```python
from build123d import *

# Parameters (mm, degrees)
EXTRUDE_1_DEPTH     = 7
SKETCH_2_R          = 15
EXTRUDE_2_DEPTH     = 18.4
EXTRUDE_3_DEPTH     = 7
EXTRUDE_START       = 6.3
SKETCH_4_R          = 15
EXTRUDE_4_DEPTH     = 6.3
SKETCH_5_R          = 15
EXTRUDE_5_DEPTH     = 6.3
SKETCH_6_R          = 5
CUT_EXTRUDE_1_DEPTH = 90.291681756


with BuildPart() as part:
    # 草图1 → 凸台-拉伸1 (new body)
    with BuildSketch(Plane.XY.offset(28.9)):
        with BuildLine():
            Line((42.411201909, 45.77806603), (42.129389286, 47.376304833))
            ThreePointArc((42.129389286, 47.376304833), (40.514502568, 47.409839327), (38.89961585, 47.376304833))
            Line((38.89961585, 47.376304833), (38.617803227, 45.77806603))
            ThreePointArc((38.617803227, 45.77806603), (37.528159676, 43.541003491), (35.420005537, 42.219088972))
            ThreePointArc((35.420005537, 42.219088972), (32.937471152, 42.04939837), (30.741018632, 43.218743572))
            Line((30.741018632, 43.218743572), (29.573606233, 44.346100621))
            ThreePointArc((29.573606233, 44.346100621), (28.247424353, 43.424024), (26.960664635, 42.447687427))
            Line((26.960664635, 42.447687427), (27.672094632, 40.98903977))
            ThreePointArc((27.672094632, 40.98903977), (28.10546685, 38.538741749), (27.176936184, 36.230148526))
            ThreePointArc((27.176936184, 36.230148526), (25.268265311, 34.633668845), (22.80397403, 34.288646587))
            Line((22.80397403, 34.288646587), (21.196873713, 34.514509808))
            ThreePointArc((21.196873713, 34.514509808), (20.665953073, 32.989024), (20.198818833, 31.442812735))
            Line((20.198818833, 31.442812735), (21.631749371, 30.680910052))
            ThreePointArc((21.631749371, 30.680910052), (23.422603901, 28.95330711), (24.028363863, 26.539839327))
            ThreePointArc((24.028363863, 26.539839327), (23.422603901, 24.126371544), (21.631749371, 22.398768602))
            Line((21.631749371, 22.398768602), (20.198818833, 21.63686592))
            ThreePointArc((20.198818833, 21.63686592), (20.665953073, 20.090654655), (21.196873713, 18.565168847))
            Line((21.196873713, 18.565168847), (22.80397403, 18.791032067))
            ThreePointArc((22.80397403, 18.791032067), (25.268265311, 18.446009809), (27.176936184, 16.849530129))
            ThreePointArc((27.176936184, 16.849530129), (28.10546685, 14.540936905), (27.672094632, 12.090638884))
            Line((27.672094632, 12.090638884), (26.960664635, 10.631991228))
            ThreePointArc((26.960664635, 10.631991228), (28.247424353, 9.655654655), (29.573606233, 8.733578033))
            Line((29.573606233, 8.733578033), (30.741018632, 9.860935083))
            ThreePointArc((30.741018632, 9.860935083), (32.937471152, 11.030280285), (35.420005536, 10.860589683))
            ThreePointArc((35.420005536, 10.860589683), (37.528159676, 9.538675164), (38.617803227, 7.301612625))
            Line((38.617803227, 7.301612625), (38.89961585, 5.703373822))
            ThreePointArc((38.89961585, 5.703373822), (40.514502568, 5.669839327), (42.129389286, 5.703373822))
            Line((42.129389286, 5.703373822), (42.411201909, 7.301612625))
            ThreePointArc((42.411201909, 7.301612625), (43.50084546, 9.538675164), (45.6089996, 10.860589683))
            ThreePointArc((45.6089996, 10.860589683), (48.091533984, 11.030280285), (50.287986504, 9.860935083))
            Line((50.287986504, 9.860935083), (51.455398903, 8.733578033))
            ThreePointArc((51.455398903, 8.733578033), (52.781580783, 9.655654655), (54.068340501, 10.631991228))
            Line((54.068340501, 10.631991228), (53.356910504, 12.090638884))
            ThreePointArc((53.356910504, 12.090638884), (52.923538286, 14.540936905), (53.852068952, 16.849530129))
            ThreePointArc((53.852068952, 16.849530129), (55.760739826, 18.446009809), (58.225031106, 18.791032067))
            Line((58.225031106, 18.791032067), (59.832131424, 18.565168847))
            ThreePointArc((59.832131424, 18.565168847), (60.363052063, 20.090654655), (60.830186304, 21.63686592))
            Line((60.830186304, 21.63686592), (59.397255765, 22.398768602))
            ThreePointArc((59.397255765, 22.398768602), (57.606401235, 24.126371544), (57.000641274, 26.539839327))
            ThreePointArc((57.000641274, 26.539839327), (57.606401235, 28.95330711), (59.397255765, 30.680910052))
            Line((59.397255765, 30.680910052), (60.830186304, 31.442812735))
            ThreePointArc((60.830186304, 31.442812735), (60.363052063, 32.989024), (59.832131424, 34.514509808))
            Line((59.832131424, 34.514509808), (58.225031106, 34.288646587))
            ThreePointArc((58.225031106, 34.288646587), (55.760739826, 34.633668845), (53.852068952, 36.230148526))
            ThreePointArc((53.852068952, 36.230148526), (52.923538286, 38.538741749), (53.356910504, 40.98903977))
            Line((53.356910504, 40.98903977), (54.068340501, 42.447687427))
            ThreePointArc((54.068340501, 42.447687427), (52.781580783, 43.424024), (51.455398903, 44.346100621))
            Line((51.455398903, 44.346100621), (50.287986504, 43.218743572))
            ThreePointArc((50.287986504, 43.218743572), (48.091533984, 42.04939837), (45.6089996, 42.219088972))
            ThreePointArc((45.6089996, 42.219088972), (43.50084546, 43.541003491), (42.411201909, 45.77806603))
        make_face()
    extrude(amount=-EXTRUDE_1_DEPTH)

    # 草图2 → 凸台-拉伸2 (add)
    with BuildSketch(Plane(origin=(0, 0, 21.9), x_dir=(-1, 0, 0), z_dir=(0, 0, -1))):
        with Locations((-40.514502568, 26.539839327)):
            Circle(SKETCH_2_R)
    extrude(amount=EXTRUDE_2_DEPTH)

    # 草图3 → 凸台-拉伸3 (add)
    with BuildSketch(Plane.XY.offset(3.5)):
        with BuildLine():
            Line((42.411201909, 45.77806603), (42.129389286, 47.376304833))
            ThreePointArc((42.129389286, 47.376304833), (40.514502568, 47.409839327), (38.89961585, 47.376304833))
            Line((38.89961585, 47.376304833), (38.617803227, 45.77806603))
            ThreePointArc((38.617803227, 45.77806603), (37.528159676, 43.541003491), (35.420005537, 42.219088972))
            ThreePointArc((35.420005537, 42.219088972), (32.937471152, 42.04939837), (30.741018632, 43.218743572))
            Line((30.741018632, 43.218743572), (29.573606233, 44.346100621))
            ThreePointArc((29.573606233, 44.346100621), (28.247424353, 43.424024), (26.960664635, 42.447687427))
            Line((26.960664635, 42.447687427), (27.672094632, 40.98903977))
            ThreePointArc((27.672094632, 40.98903977), (28.10546685, 38.538741749), (27.176936184, 36.230148526))
            ThreePointArc((27.176936184, 36.230148526), (25.268265311, 34.633668845), (22.80397403, 34.288646587))
            Line((22.80397403, 34.288646587), (21.196873713, 34.514509808))
            ThreePointArc((21.196873713, 34.514509808), (20.665953073, 32.989024), (20.198818833, 31.442812735))
            Line((20.198818833, 31.442812735), (21.631749371, 30.680910052))
            ThreePointArc((21.631749371, 30.680910052), (23.422603901, 28.95330711), (24.028363863, 26.539839327))
            ThreePointArc((24.028363863, 26.539839327), (23.422603901, 24.126371544), (21.631749371, 22.398768602))
            Line((21.631749371, 22.398768602), (20.198818833, 21.63686592))
            ThreePointArc((20.198818833, 21.63686592), (20.665953073, 20.090654655), (21.196873713, 18.565168847))
            Line((21.196873713, 18.565168847), (22.80397403, 18.791032067))
            ThreePointArc((22.80397403, 18.791032067), (25.268265311, 18.446009809), (27.176936184, 16.849530129))
            ThreePointArc((27.176936184, 16.849530129), (28.10546685, 14.540936905), (27.672094632, 12.090638884))
            Line((27.672094632, 12.090638884), (26.960664635, 10.631991228))
            ThreePointArc((26.960664635, 10.631991228), (28.247424353, 9.655654655), (29.573606233, 8.733578033))
            Line((29.573606233, 8.733578033), (30.741018632, 9.860935083))
            ThreePointArc((30.741018632, 9.860935083), (32.937471152, 11.030280285), (35.420005536, 10.860589683))
            ThreePointArc((35.420005536, 10.860589683), (37.528159676, 9.538675164), (38.617803227, 7.301612625))
            Line((38.617803227, 7.301612625), (38.89961585, 5.703373822))
            ThreePointArc((38.89961585, 5.703373822), (40.514502568, 5.669839327), (42.129389286, 5.703373822))
            Line((42.129389286, 5.703373822), (42.411201909, 7.301612625))
            ThreePointArc((42.411201909, 7.301612625), (43.50084546, 9.538675164), (45.6089996, 10.860589683))
            ThreePointArc((45.6089996, 10.860589683), (48.091533984, 11.030280285), (50.287986504, 9.860935083))
            Line((50.287986504, 9.860935083), (51.455398903, 8.733578033))
            ThreePointArc((51.455398903, 8.733578033), (52.781580783, 9.655654655), (54.068340501, 10.631991228))
            Line((54.068340501, 10.631991228), (53.356910504, 12.090638884))
            ThreePointArc((53.356910504, 12.090638884), (52.923538286, 14.540936905), (53.852068952, 16.849530129))
            ThreePointArc((53.852068952, 16.849530129), (55.760739826, 18.446009809), (58.225031106, 18.791032067))
            Line((58.225031106, 18.791032067), (59.832131424, 18.565168847))
            ThreePointArc((59.832131424, 18.565168847), (60.363052063, 20.090654655), (60.830186304, 21.63686592))
            Line((60.830186304, 21.63686592), (59.397255765, 22.398768602))
            ThreePointArc((59.397255765, 22.398768602), (57.606401235, 24.126371544), (57.000641274, 26.539839327))
            ThreePointArc((57.000641274, 26.539839327), (57.606401235, 28.95330711), (59.397255765, 30.680910052))
            Line((59.397255765, 30.680910052), (60.830186304, 31.442812735))
            ThreePointArc((60.830186304, 31.442812735), (60.363052063, 32.989024), (59.832131424, 34.514509808))
            Line((59.832131424, 34.514509808), (58.225031106, 34.288646587))
            ThreePointArc((58.225031106, 34.288646587), (55.760739826, 34.633668845), (53.852068952, 36.230148526))
            ThreePointArc((53.852068952, 36.230148526), (52.923538286, 38.538741749), (53.356910504, 40.98903977))
            Line((53.356910504, 40.98903977), (54.068340501, 42.447687427))
            ThreePointArc((54.068340501, 42.447687427), (52.781580783, 43.424024), (51.455398903, 44.346100621))
            Line((51.455398903, 44.346100621), (50.287986504, 43.218743572))
            ThreePointArc((50.287986504, 43.218743572), (48.091533984, 42.04939837), (45.6089996, 42.219088972))
            ThreePointArc((45.6089996, 42.219088972), (43.50084546, 43.541003491), (42.411201909, 45.77806603))
        make_face()
    extrude(amount=-EXTRUDE_3_DEPTH)

    # 草图4 → 凸台-拉伸4 (add)
    with BuildSketch(Plane.XY.offset(28.9).offset(EXTRUDE_START)):
        with Locations(Location((40.514502568, 26.539839327, 0), (0, 0, 180))):
            Circle(SKETCH_4_R)
    extrude(amount=-EXTRUDE_4_DEPTH)

    # 草图5 → 凸台-拉伸5 (add)
    with BuildSketch(Plane(origin=(0, 0, -3.5), x_dir=(-1, 0, 0), z_dir=(0, 0, -1))):
        with Locations((-40.514502568, 26.539839327)):
            Circle(SKETCH_5_R)
    extrude(amount=EXTRUDE_5_DEPTH)

    # 草图6 → 切除-拉伸1 (cut, through all)
    with BuildSketch(Plane(origin=(0, 0, -9.8), x_dir=(-1, 0, 0), z_dir=(0, 0, -1))):
        with Locations((-40.514502568, 26.539839327)):
            Circle(SKETCH_6_R)
    extrude(amount=-CUT_EXTRUDE_1_DEPTH, mode=Mode.SUBTRACT)


solid = part.part
```
Design review of the part built by this model. Coordinates are the model's own, in mm. A direction names the side the tool comes from. Coordinates: 2 decimals unless noted, no trailing zeros. Order: outer loops, then holes, each group sorted by start corner. A loop starts at its lowest first (then second) coordinate and runs counter-clockwise, first axis right, second up. Notation, with made-up numbers: (48, 7.5) -> (65, 7.5) arc R7 cw to (65, 17.5) -> close; hole circle Ø2 at (53, 38.25). An arc over 180 degrees is marked (long way). One line per item, written item: value. Start each with the question number.
Q1. Take a section at B-B, the plane y = 28.5. State the section outline as (x, z) points.
Q2. Take a section at A-A, the plane x = 41. State the section outline as (y, z) points, then the cut area to 3 significant figures.
Q3. For probe 1 along Y at (x, z) = (40.5, 13.5); probe 2 along X at (y, z) = (9.5, 27.5); probe 3 along X at (y, z) = (29, 8), list the stretches that pass through material, from the lowest coordinate up.
Q4. Tool access review of faces 5 (the flat face through (22, 34.4, 0)), 6 (the flat face through (30.15, 9.29, 0.05)), 7 (the flat face through (53.71, 41.71, 25.45)): name each direction out of +Z, -Z, +X, -X, +Y, -Y from which nothing blocks a thin tool from reaching the whole face with its end or side.
Q5. Take a section at C-C, the plane z = 10.5. State the section outline as (x, y) points.
Q6. Mouldability with a two-part tool opening along X and no side actions: class faces 1 (the flat face through (49.45, 14.27, 28.9)), 2 (the cylindrical face through (32.903, 11.023, 25.449)), 3 (the cylindrical face through (52.76, 9.64, 25.45)), 4 (the cylindrical face through (28.11, 38.57, 0.05)) as pulls with the +X half, pulls with the -X half, needs draft (parallel to the pull), parting line crosses it, or undercut.
Q7. Take a section at D-D, the plane x = 49. State the section outline as (y, z) points, then the cut area to 3 significant figures.
Q8. Insertion check: pin 1 Ø3 at (x, z) = (49, 7) entering from -Y; pin 2 Ø1 at (x, y) = (56.5, 20.5) entering from -Z; pin 3 Ø1.5 at (y, z) = (33, 8.5) entering from -X; pin 4 Ø11.5 at (x, y) = (40.51, 26.54) entering from -Z. Each pin has a flat end and moves straight along its axis. Give the tip position at first contact, or say it passes through.
Values follow:
1. outline: (23.65, -3.5) -> (25.64, -3.5) -> (25.64, -9.8) -> (35.91, -9.8) -> (35.91, 35.2) -> (25.64, 35.2) -> (25.64, 28.9) -> (23.65, 28.9) -> (23.65, 21.9) -> (25.64, 21.9) -> (25.64, 3.5) -> (23.65, 3.5) -> close; (45.11, -9.8) -> (55.39, -9.8) -> (55.39, -3.5) -> (57.38, -3.5) -> (57.38, 3.5) -> (55.39, 3.5) -> (55.39, 21.9) -> (57.38, 21.9) -> (57.38, 28.9) -> (55.39, 28.9) -> (55.39, 35.2) -> (45.11, 35.2) -> close
2. outline: (5.67, -3.5) -> (11.55, -3.5) -> (11.55, -9.8) -> (21.56, -9.8) -> (21.56, 35.2) -> (11.55, 35.2) -> (11.55, 28.9) -> (5.67, 28.9) -> (5.67, 21.9) -> (11.55, 21.9) -> (11.55, 3.5) -> (5.67, 3.5) -> close; (31.52, -9.8) -> (41.53, -9.8) -> (41.53, -3.5) -> (47.41, -3.5) -> (47.41, 3.5) -> (41.53, 3.5) -> (41.53, 21.9) -> (47.41, 21.9) -> (47.41, 28.9) -> (41.53, 28.9) -> (41.53, 35.2) -> (31.52, 35.2) -> close
2. area: 1,070 mm2
3. probe 1: y = 11.54 to 21.54, 31.54 to 41.54
3. probe 2: x = 28.46 to 30.37, 37.56 to 43.47, 50.66 to 52.57
3. probe 3: x = 25.72 to 36.16, 44.87 to 55.31
4. face 5: +Z, -Z, +Y
4. face 6: +Z, -Z, -Y
4. face 7: +Z, -Z, +X
5. outline: circle Ø30 at (40.51, 26.54); hole circle Ø10 at (40.51, 26.54)
6. face 1: needs draft
6. face 2: undercut
6. face 3: pulls with the +X half
6. face 4: pulls with the -X half
7. outline: (10.73, -3.5) -> (14.17, -3.5) -> (14.17, -9.8) -> (38.91, -9.8) -> (38.91, -3.5) -> (42.35, -3.5) -> (42.35, 3.5) -> (38.91, 3.5) -> (38.91, 21.9) -> (42.35, 21.9) -> (42.35, 28.9) -> (38.91, 28.9) -> (38.91, 35.2) -> (14.17, 35.2) -> (14.17, 28.9) -> (10.73, 28.9) -> (10.73, 21.9) -> (14.17, 21.9) -> (14.17, 3.5) -> (10.73, 3.5) -> close
7. area: 1,210 mm2
8. pin 1: stops at y = 13.27
8. pin 2: stops at z = -3.5
8. pin 3: stops at x = 26.64
8. pin 4: stops at z = -9.8
